Verification items for this drawing (mm, ordinates from the low corner). Give positions to 0.01 mm unless a question says otherwise; leave off trailing zeros. Write each loop counter-clockwise with the first axis right and the second up, starting at its lowest first coordinate (ties: lowest second). Pieces come first, ordered by that corner, then holes. Notation, with made-up numbers: M 3,7.5 L 53,7.5 A9 ccw 53,23.5 Z; hole C -25,67.5 d9. An arc over 180 degrees is marked long. Use one line per item in the form item = value. Start each with the question number.
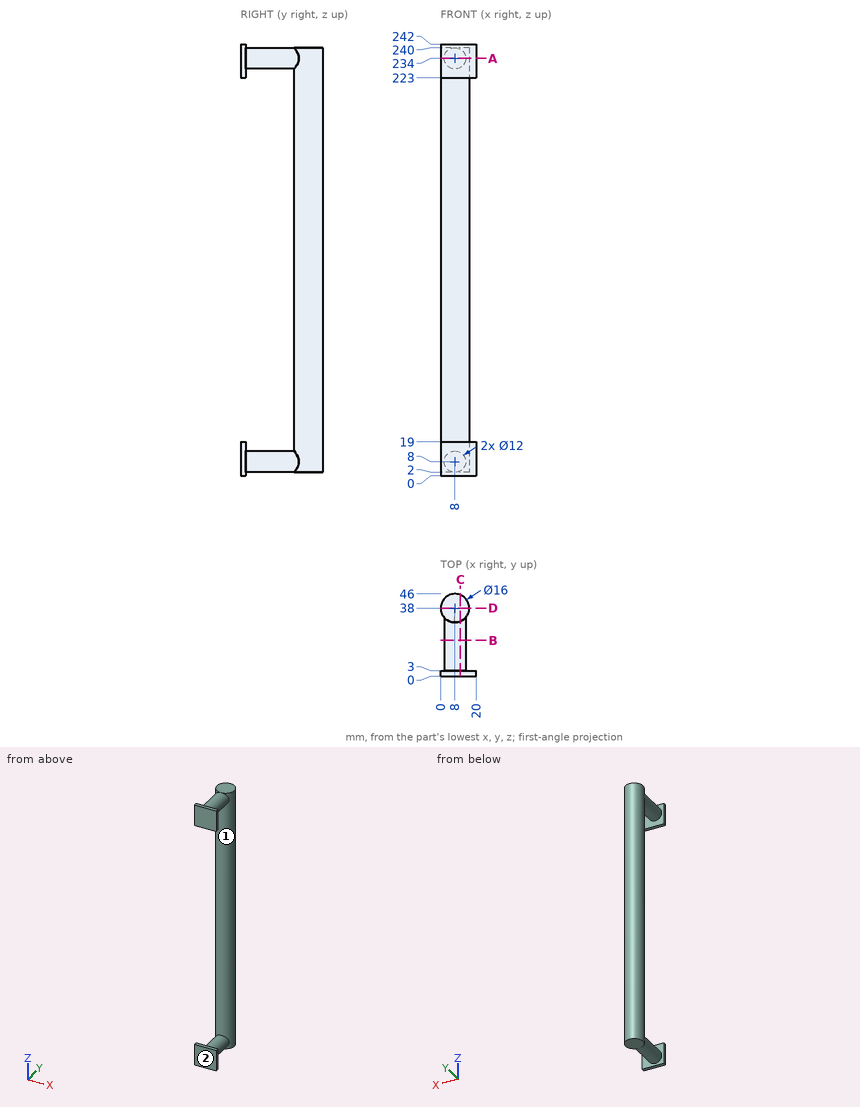
(1) Sectioned sample at A-A, the plane z = 234. Record the boundary of the cut face in (x, y).
(2) Sectioned sample at D-D, the plane y = 38. Record the boundary of the cut face in (x, z).
(3) Depth check by flat-ended pin: pin 1 (12 mm diameter, centred on x = 3, z = 87, fed in from +Y); pin 2 (12 mm diameter, centred on x = 7.5, y = 11, fed in from +Z); pin 3 (12 mm diameter, centred on y = 29, z = 61, fed in from +X); pin 4 (8 mm diameter, centred on x = 8.5, y = 37, fed in from -Z). Enter the tip coordinate at first touch or a pass-through.
(4) Sectioned sample at B-B, the plane y = 20. Record the boundary of the cut face in (x, z), plus the area to 3 significant figures.
(5) Draft check along Z on the marked faces 1 and 2. Enter one of: released by +Z, released by -Z, zero draft, split by the parting line, or undercut.
(6) Sectioned sample at C-C, the plane x = 11. Record the boundary of the cut face in (y, z).
(7) Thickness scan on probe 1 along Z at (x, y) = (7.25, 40); probe 2 along Z at (x, y) = (10.25, 4); probe 3 along Z at (x, y) = (5.25, 29.5). Record the ranges inside material, lowest first. Write a range as [from, to].
Numbers:
q1.outline = M 0,0 L 20,0 L 20,3 L 14,3 L 14,32.71 A8 ccw long 2,32.71 L 2,3 L 0,3 Z
q2.outline = M 0,2 L 16,2 L 16,240 L 0,240 Z
q3.pin_1 = 46
q3.pin_2 = 240
q3.pin_3 = 15.42
q3.pin_4 = 2
q4.outline = C 8,8 d12; C 8,234 d12
q4.area = 226 mm2
q5.face_1 = undercut
q5.face_2 = zero draft
q6.outline = M 0,0 L 3,0 L 3,2.8 L 30.58,2.8 L 30.58,2 L 45.42,2 L 45.42,240 L 30.58,240 L 30.58,239.2 L 3,239.2 L 3,242 L 0,242 L 0,223 L 3,223 L 3,228.8 L 30.58,228.8 L 30.58,13.2 L 3,13.2 L 3,19 L 0,19 Z
q7.probe_1 = [2, 240]
q7.probe_2 = [2.44, 13.56], [228.44, 239.56]
q7.probe_3 = [2.67, 13.33], [228.67, 239.33]
